Study the drawing (mm; zero at the part's minimum x, y, z) and answer. A direction names the side the tool comes from. Round coordinates to 2 decimals unless told otherwise and drop trailing zeros. Order: outer loops, then holes, each group sorted by start corner. A loop starts at its lowest first (then second) coordinate and runs counter-clockwise, first axis right, second up. Notation, with made-up numbers: M 24.25,34 L 29.25,34 A12 cw 29.25,53 Z; hole C -35.75,-20 d1. An arc over 180 degrees is marked long. Put each result on its own line as item: value. Start each with the question number.
1. The part is cut by section A-A (x = 5). Give the vertices of the cut face in (y, z).
2. The part is cut by section B-B (z = 0.55). Give the vertices of the cut face in (x, y) (1 decimal).
3. Each of these flat-tipped pins is pushed along its axis until it touches: pin 1 Ø1.5 at (x, y) = (5, 6) entering from -Z; pin 2 Ø0.5 at (x, z) = (18.5, 0.5) entering from +Y; pin 3 Ø0.5 at (x, z) = (19, 0.5) entering from -Y. Where does it stop, or does it pass through?
4. The part is cut by section C-C (y = 5). Give the vertices of the cut face in (x, z) (1 decimal).
5. The mould has two halves that part along X. Classify the marked faces 3, 4 and 5: +X half, -X half, draft (parallel to the pull), parting line (faces both ways), or undercut.
6. The part is cut by section D-D (x = 12). Give the vertices of the cut face in (y, z).
7. Which of the six approach directions +Z, -Z, +X, -X, +Y, -Y give full straight-line access (tool end or side, diameter ignored) to the marked faces 1 and 2?
8. Consider line 1 (Y direction, x = 5, z = 0.9); line 2 (Y direction, x = 15.5, z = 0.9); line 3 (X direction, y = 4.5, z = 1.4) (1 decimal). Determine where each line is inside the solid, lowest interval first.
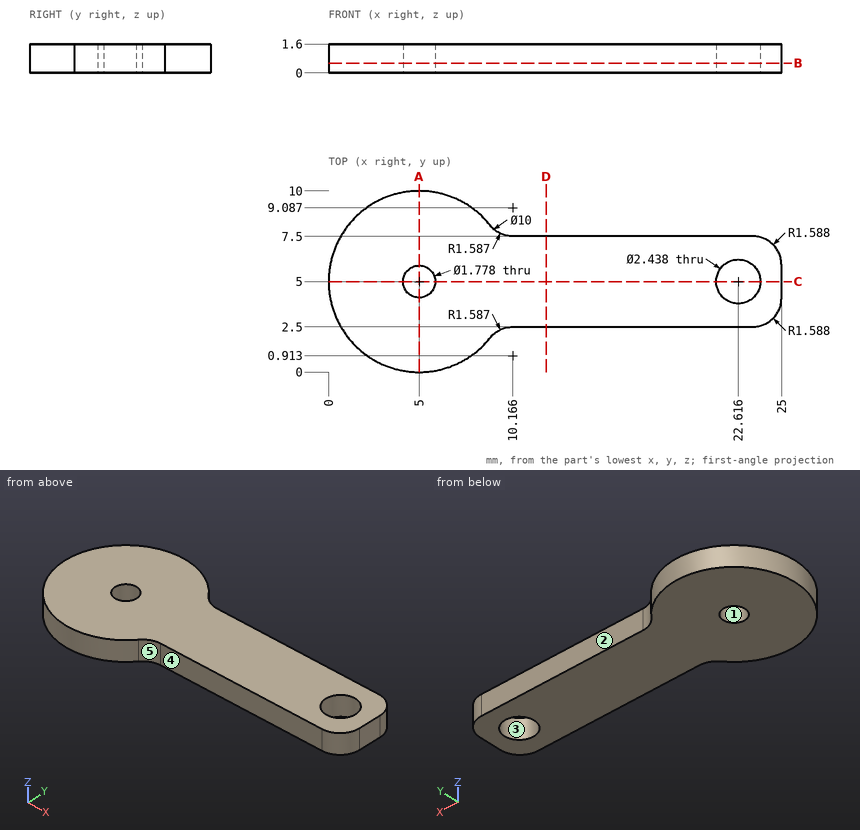
Resolved:
1. outline: M 0,0 L 4.11,0 L 4.11,1.6 L 0,1.6 Z; M 5.89,0 L 10,0 L 10,1.6 L 5.89,1.6 Z
2. outline: M 8.9,1.9 A1.6 cw 10.2,2.5 L 23.4,2.5 A1.6 ccw 25,4.1 L 25,5.9 A1.6 ccw 23.4,7.5 L 10.2,7.5 A1.6 cw 8.9,8.1 A5 ccw long Z; hole C 5,5 d1.8; hole C 22.6,5 d2.4
3. pin 1: z = 0
3. pin 2: y = 7.5
3. pin 3: y = 2.5
4. outline: M 0,0 L 4.1,0 L 4.1,1.6 L 0,1.6 Z; M 5.9,0 L 21.4,0 L 21.4,1.6 L 5.9,1.6 Z; M 23.8,0 L 25,0 L 25,1.6 L 23.8,1.6 Z
5. face 3: undercut
5. face 4: draft
5. face 5: +X half
6. outline: M 2.5,0 L 7.5,0 L 7.5,1.6 L 2.5,1.6 Z
7. face 1: +Z, -Z
7. face 2: +Z, -Z, +X, +Y
8. line 1: 0 to 4.11, 5.89 to 10
8. line 2: 2.5 to 7.5
8. line 3: 0 to 4.3, 5.7 to 21.5, 23.7 to 25
